```python
from build123d import *

# Parameters (mm, degrees)
F0_R     = 50.8
F1_DEPTH = 25.4
F2_R     = 49.149
F3_DEPTH = 6.35
F4_R     = 46.355
F5_DEPTH = 27.94
F7_DEPTH = 31.751
F9_DEPTH = 2.54
F10_SIZE = 0.762


with BuildPart() as f1:
    # F0 (on Top) → F1 (new body)
    with BuildSketch(Plane.XY):
        Circle(F0_R)
    extrude(amount=F1_DEPTH)

    # F2 (on face) → F3 (join)
    with BuildSketch(Plane.XY.offset(25.4)):
        Circle(F2_R)
    extrude(amount=F3_DEPTH)

    # F4 (on face) → F5 (cut)
    with BuildSketch(Plane.XY.offset(31.75)):
        Circle(F4_R)
    extrude(amount=-F5_DEPTH, mode=Mode.SUBTRACT)

    # F6 (on face) → F7 (cut, through all)
    with BuildSketch(Plane(origin=(0, 0, 0), x_dir=(1, 0, 0), z_dir=(0, 0, -1))):
        with BuildLine():
            ThreePointArc((26.263693, 18.529348), (21.249092, 24.116268), (15.075286, 28.387569))
            Line((15.075286, 28.387569), (12.097015, 22.779325))
            ThreePointArc((12.097015, 22.779325), (17.051125, 19.351862), (21.075042, 14.868693))
            Line((21.075042, 14.868693), (26.263693, 18.529348))
        make_face()
        with BuildLine():
            ThreePointArc((-18.529348, 26.263693), (-24.116268, 21.249092), (-28.387569, 15.075286))
            Line((-28.387569, 15.075286), (-22.779325, 12.097015))
            ThreePointArc((-22.779325, 12.097015), (-19.351862, 17.051125), (-14.868693, 21.075042))
            Line((-14.868693, 21.075042), (-18.529348, 26.263693))
        make_face()
        with BuildLine():
            ThreePointArc((-26.263693, -18.529348), (-21.249092, -24.116268), (-15.075286, -28.387569))
            Line((-15.075286, -28.387569), (-12.097015, -22.779325))
            ThreePointArc((-12.097015, -22.779325), (-17.051125, -19.351862), (-21.075042, -14.868693))
            Line((-21.075042, -14.868693), (-26.263693, -18.529348))
        make_face()
        with BuildLine():
            ThreePointArc((18.529348, -26.263693), (24.116268, -21.249092), (28.387569, -15.075286))
            Line((28.387569, -15.075286), (22.779325, -12.097015))
            ThreePointArc((22.779325, -12.097015), (19.351862, -17.051125), (14.868693, -21.075042))
            Line((14.868693, -21.075042), (18.529348, -26.263693))
        make_face()
    extrude(amount=-F7_DEPTH, mode=Mode.SUBTRACT)

    # F8 (on face) → F9 (cut)
    with BuildSketch(Plane.XY.offset(3.81)):
        with BuildLine():
            Line((-22.118151, 13.267361), (-27.563613, 16.533769))
            ThreePointArc((-27.563613, 16.533769), (-28.329177, 15.184731), (-29.028766, 13.800328))
            Line((-29.028766, 13.800328), (-23.293849, 11.073938))
            ThreePointArc((-23.293849, 11.073938), (-22.73247, 12.184838), (-22.118151, 13.267361))
        make_face()
        with BuildLine():
            Line((-13.267361, -22.118151), (-16.533769, -27.563613))
            ThreePointArc((-16.533769, -27.563613), (-15.184731, -28.329177), (-13.800328, -29.028766))
            Line((-13.800328, -29.028766), (-11.073938, -23.293849))
            ThreePointArc((-11.073938, -23.293849), (-12.184838, -22.73247), (-13.267361, -22.118151))
        make_face()
        with BuildLine():
            Line((22.118151, -13.267361), (27.563613, -16.533769))
            ThreePointArc((27.563613, -16.533769), (28.329177, -15.184731), (29.028766, -13.800328))
            Line((29.028766, -13.800328), (23.293849, -11.073938))
            ThreePointArc((23.293849, -11.073938), (22.73247, -12.184838), (22.118151, -13.267361))
        make_face()
        with BuildLine():
            Line((13.267361, 22.118151), (16.533769, 27.563613))
            ThreePointArc((16.533769, 27.563613), (15.184731, 28.329177), (13.800328, 29.028766))
            Line((13.800328, 29.028766), (11.073938, 23.293849))
            ThreePointArc((11.073938, 23.293849), (12.184838, 22.73247), (13.267361, 22.118151))
        make_face()
    extrude(amount=-F9_DEPTH, mode=Mode.SUBTRACT)

    # F10
    f10_edges = [f1.edges().sort_by_distance(p)[0] for p in [
        (-23.669367, 16.69902, 3.81),
        (-24.840882, 14.900565, 3.81),
        (12.437133, 26.161307, 3.81),
        (14.900565, 24.840882, 3.81),
        (24.840882, -14.900565, 3.81),
        (26.161307, -12.437133, 3.81),
        (-12.437133, -26.161307, 3.81),
        (-14.900565, -24.840882, 3.81),
        (23.669367, -16.69902, 3.81),
        (16.69902, 23.669367, 3.81),
        (-16.69902, -23.669367, 3.81),
    ]]
    chamfer(f10_edges, length=F10_SIZE)


solid = f1.part
```
Geometry: final body of the model. Coordinates: model frame, mm. A direction names the side the tool comes from. Round coordinates to 2 decimals unless told otherwise and drop trailing zeros. Write each loop counter-clockwise with the first axis right and the second up, starting at its lowest first coordinate (ties: lowest second). Pieces come first, ordered by that corner, then holes.
Item 1: Material intervals for L1, parallel to Y at x = 0, z = 26 (3 decimals); L2, parallel to Y at x = -14, z = 2.5; L3, parallel to Y at x = 0, z = 14 (3 decimals), sorted ascending.
Item 2: Set-up query: faces 3 (the face through (15.213, 28.314, 2.558)), 4 (the face through (25.623, 13.607, 1.878)). Return all of +Z, -Z, +X, -X, +Y, -Y with unobstructed straight access to the full face (end or side cutting, diameter ignored); none if empty.
Item 3: Section query C-C (z = 7.5). Return loops of the section in (x, y) (3 decimals), plus the area to 3 significant figures.
Item 4: Mould query, pull axis X, two halves, no side actions, for faces 1 (the face through (14, 26, 1.27)), 2 (the face through (-11.012, -49.592, 12.522)). Classes: +X half, -X half, draft (parallel to the pull), parting line (faces both ways), or undercut.
Item 5: Pin query (flat end, axial travel): P1, Ø4.5, axis at x = 14.5, y = 26.5, coming from the +Z side; P2, Ø1.5, axis at x = -8.5, z = 4.5, coming from the +Y side; P3, Ø10, axis at y = 38, z = 9, coming from the -X side. Return the tip coordinate at first contact, or that it passes through.
Item 6: Section query A-A (x = 0). Return loops of the section in (y, z) (3 decimals), plus the area to 3 significant figures.
Completed:
1. L1: y = -49.149 to -46.355, 46.355 to 49.149
1. L2: y = -48.83 to -28.93, -23.34 to 21.66, 26.36 to 48.83
1. L3: y = -50.8 to -46.355, 46.355 to 50.8
2. face 3: +Z
2. face 4: +Z, -Z
3. outline: circle Ø101.6 at (0, 0); hole circle Ø92.71 at (0, 0)
3. area: 1,360 mm2
4. face 1: undercut
4. face 2: parting line
5. P1: stops at z = 3.81
5. P2: stops at y = 50.21
5. P3: stops at x = -38.62
6. outline: (-50.8, 0) - (50.8, 0) - (50.8, 25.4) - (49.149, 25.4) - (49.149, 31.75) - (46.355, 31.75) - (46.355, 3.81) - (-46.355, 3.81) - (-46.355, 31.75) - (-49.149, 31.75) - (-49.149, 25.4) - (-50.8, 25.4) - close
6. area: 615 mm2
